from build123d import *

# Parameters (mm, degrees)
F0_W     = 40
F0_H     = 68
F0_W_2   = 36
F0_H_2   = 64
F1_DEPTH = 20
F2_DEPTH = 15
F3_W     = 10
F3_H     = 5
F4_DEPTH = 25
F5_W     = 26
F5_H     = 54
F6_DEPTH = 2
F7_W     = 7.968329
F7_H     = 7
F8_DEPTH = 7
F9_R     = 3


with BuildPart() as f1:
    # F0 (on Top) → F1 (new body)
    with BuildSketch(Plane.XY):
        Rectangle(F0_W, F0_H)
        Rectangle(F0_W_2, F0_H_2, mode=Mode.SUBTRACT)
        Rectangle(F0_W_2, F0_H_2)
    extrude(amount=F1_DEPTH)

    # F0 (on Top) → F2 (cut)
    with BuildSketch(Plane.XY):
        Rectangle(F0_W_2, F0_H_2)
    extrude(amount=F2_DEPTH, mode=Mode.SUBTRACT)

    # F3 (on face) → F4 (cut)
    with BuildSketch(Plane(origin=(0, 34, 0), x_dir=(-1, 0, 0), z_dir=(0, 1, 0))):
        with Locations((10.149879, 2.5)):
            Rectangle(F3_W, F3_H)
    extrude(amount=-F4_DEPTH, mode=Mode.SUBTRACT)

    # F5 (on face) → F6 (join)
    with BuildSketch(Plane(origin=(0, 0, 0), x_dir=(1, 0, 0), z_dir=(0, 0, -1))):
        Polygon((20, 34), (-20, 34), (-20, -34), (-15.149879, -34), (-15.149879, -32), (-18, -32), (-18, 32), (18, 32), (18, -32), (-5.149879, -32), (-5.149879, -34), (20, -34), align=None)
        Polygon((-15.149879, -32), (-15.149879, -34), (-5.149879, -34), (-5.149879, -32), (18, -32), (18, 32), (-18, 32), (-18, -32), align=None)
        Rectangle(F5_W, F5_H, mode=Mode.SUBTRACT)
    extrude(amount=F6_DEPTH)

    # F7 (on face) → F8 (cut)
    with BuildSketch(Plane(origin=(0, 0, -2), x_dir=(1, 0, 0), z_dir=(0, 0, -1))):
        with Locations((-9.015835, -30.5)):
            Rectangle(F7_W, F7_H)
    extrude(amount=-F8_DEPTH, mode=Mode.SUBTRACT)

    # F9
    f9_edges = [f1.edges().sort_by_distance(p)[0] for p in [
        (-20, 0, 20),
        (0, -34, 20),
        (20, 0, 20),
        (0, 34, 20),
        (20, 34, 9),
        (-20, -34, 9),
        (-20, 0, -2),
        (-20, 34, 9),
        (20, -34, 9),
        (20, 0, -2),
        (0, -34, -2),
        (7.484165, 34, -2),
    ]]
    fillet(f9_edges, radius=F9_R)


solid = f1.part
Could you check a few things on this model? Use its own coordinates, in mm. A direction names the side the tool comes from. Round coordinates to 2 decimals unless told otherwise and drop trailing zeros. Write each loop counter-clockwise with the first axis right and the second up, starting at its lowest first coordinate (ties: lowest second). Pieces come first, ordered by that corner, then holes. Notation, with made-up numbers: (74, -29) - (125, -29) arc R23 ccw to (125, -8) - close; hole circle Ø11 at (64, 86). An arc over 180 degrees is marked (long way). Put each result on its own line as item: value. Start each with the question number.
(1) For faces 1 (the flat face through (13, 0, -1)), 2 (the flat face through (-18, 0, 7)), 3 (the flat face through (-15.15, 33, 2)), 4 (the flat face through (-5.032, 33, 1)), which set-ups out of +Z, -Z, +X, -X, +Y, -Y let a thin tool reach every point of the face, with its end or its side?
(2) I need wall thicknesses on probe 1 along X at (y, z) = (23.5, 8.75); probe 2 along Z at (x, y) = (-16.5, -27); probe 3 along Y at (x, z) = (-2.5, 13.75). Which ranges of each line are inside material? Lowest first, please.
(3) Thinking about a two-plate mould opening in Z: for faces 5 (the cylindrical face through (-19.1, -33.14, 8.89)), 6 (the flat face through (-10, 33, 5)), 7 (the cylindrical face through (0.24, -33.14, 19.1)), which applies, released by +Z, released by -Z, zero draft, split by the parting line, or undercut?
(4) I want a section at D-D, the plane x = -11.5. Please give me the cut outline in (y, z).
(5) I want a section at C-C, the plane y = 29. Please give me the cut outline in (x, z).
(6) I want a section at B-B, the plane x = 6. Please give me the cut outline in (y, z), plus the area to 3 significant figures.
(7) I want a section at A-A, the plane z = 13. Please give me the cut outline in (x, y), plus the area to 3 significant figures.
(8) Will these pins go through, and if not, where does the flat tip stop? pin 1 (0.6 mm diameter, centred on y = 9.5, z = -1.5, fed in from -X); pin 2 (1.6 mm diameter, centred on y = 12.5, z = -1.5, fed in from +X); pin 3 (2 mm diameter, centred on x = 6, z = -1, fed in from -Y); pin 4 (2 mm diameter, centred on y = 11.5, z = 17.5, fed in from -X).
Here are the results:
1. face 1: -Z
1. face 2: none
1. face 3: +Y
1. face 4: -Z, +Y
2. probe 1: x = -20 to -18, 18 to 20
2. probe 2: z = -2 to 0, 15 to 20
2. probe 3: y = -34 to -32, 32 to 34
3. face 5: zero draft
3. face 6: undercut
3. face 7: released by +Z
4. outline: (-34, 1) arc R3 ccw to (-31, -2) - (-27, -2) - (-27, 0) - (-32, 0) - (-32, 15) - (32, 15) - (32, 5) - (34, 5) - (34, 17) arc R3 ccw to (31, 20) - (-31, 20) arc R3 ccw to (-34, 17) - close
5. outline: (-20, 1) arc R3 ccw to (-17, -2) - (-13, -2) - (-13, 0) - (-18, 0) - (-18, 15) - (18, 15) - (18, 0) - (-5.03, 0) - (-5.03, -2) - (17, -2) arc R3 ccw to (20, 1) - (20, 17) arc R3 ccw to (17, 20) - (-17, 20) arc R3 ccw to (-20, 17) - close
6. outline: (-34, 1) arc R3 ccw to (-31, -2) - (-27, -2) - (-27, 0) - (-32, 0) - (-32, 15) - (32, 15) - (32, 0) - (27, 0) - (27, -2) - (31, -2) arc R3 ccw to (34, 1) - (34, 17) arc R3 ccw to (31, 20) - (-31, 20) arc R3 ccw to (-34, 17) - close
6. area: 420 mm^2
7. outline: (-20, -31) arc R3 ccw to (-17, -34) - (17, -34) arc R3 ccw to (20, -31) - (20, 31) arc R3 ccw to (17, 34) - (-17, 34) arc R3 ccw to (-20, 31) - close; hole (-18, -32) - (18, -32) - (18, 32) - (-18, 32) - close
7. area: 408 mm^2
8. pin 1: stops at x = -19.04
8. pin 2: stops at x = 19.47
8. pin 3: stops at y = -33.83
8. pin 4: stops at x = -20
